```python
from build123d import *

# Parameters (mm, degrees)
F1_DEPTH = 3.5
F2_R     = 10
F3_DEPTH = 3.501
F4_R     = 12
F4_R_2   = 10
F5_DEPTH = 25
F6_SIZE  = 1.5


with BuildPart() as f1:
    # F0 (on Top) → F1 (new body)
    with BuildSketch(Plane.XY):
        with BuildLine():
            ThreePointArc((102.5, 82.5), (96.6421356237, 96.6421356237), (82.5, 102.5))
            Line((82.5, 102.5), (-82.5, 102.5))
            ThreePointArc((-82.5, 102.5), (-96.6421356237, 96.6421356237), (-102.5, 82.5))
            Line((-102.5, 82.5), (-102.5, -82.5))
            ThreePointArc((-102.5, -82.5), (-96.6421356237, -96.6421356237), (-82.5, -102.5))
            Line((-82.5, -102.5), (82.5, -102.5))
            ThreePointArc((82.5, -102.5), (96.6421356237, -96.6421356237), (102.5, -82.5))
            Line((102.5, -82.5), (102.5, 82.5))
        make_face()
    extrude(amount=F1_DEPTH)

    # F2 (on Top) → F3 (cut, through all)
    with BuildSketch(Plane.XY):
        with Locations((-78, 78)):
            Circle(F2_R)
        with Locations((-78, 39)):
            Circle(F2_R)
        with Locations((-78, 0)):
            Circle(F2_R)
        with Locations((-78, -39)):
            Circle(F2_R)
        with Locations((-78, -78)):
            Circle(F2_R)
        with Locations((-39, 78)):
            Circle(F2_R)
        with Locations((-39, 39)):
            Circle(F2_R)
        with Locations((-39, 0)):
            Circle(F2_R)
        with Locations((-39, -39)):
            Circle(F2_R)
        with Locations((-39, -78)):
            Circle(F2_R)
        with Locations((0, 78)):
            Circle(F2_R)
        with Locations((0, 39)):
            Circle(F2_R)
        Circle(F2_R)
        with Locations((0, -39)):
            Circle(F2_R)
        with Locations((0, -78)):
            Circle(F2_R)
        with Locations((39, 78)):
            Circle(F2_R)
        with Locations((39, 39)):
            Circle(F2_R)
        with Locations((39, 0)):
            Circle(F2_R)
        with Locations((39, -39)):
            Circle(F2_R)
        with Locations((39, -78)):
            Circle(F2_R)
        with Locations((78, 78)):
            Circle(F2_R)
        with Locations((78, 39)):
            Circle(F2_R)
        with Locations((78, 0)):
            Circle(F2_R)
        with Locations((78, -39)):
            Circle(F2_R)
        with Locations((78, -78)):
            Circle(F2_R)
    extrude(amount=F3_DEPTH, mode=Mode.SUBTRACT)

    # F4 (on face) → F5 (join)
    with BuildSketch(Plane(origin=(0, 0, 0), x_dir=(1, 0, 0), z_dir=(0, 0, -1))):
        with Locations((-78, -78)):
            Circle(F4_R)
        with Locations((-78, -78)):
            Circle(F4_R_2, mode=Mode.SUBTRACT)
        with Locations((-78, 0)):
            Circle(F4_R)
        with Locations((-78, 0)):
            Circle(F4_R_2, mode=Mode.SUBTRACT)
        with Locations((-78, 78)):
            Circle(F4_R)
        with Locations((-78, 78)):
            Circle(F4_R_2, mode=Mode.SUBTRACT)
        with Locations((0, -78)):
            Circle(F4_R)
        with Locations((0, -78)):
            Circle(F4_R_2, mode=Mode.SUBTRACT)
        Circle(F4_R)
        Circle(F4_R_2, mode=Mode.SUBTRACT)
        with Locations((0, 78)):
            Circle(F4_R)
        with Locations((0, 78)):
            Circle(F4_R_2, mode=Mode.SUBTRACT)
        with Locations((78, -78)):
            Circle(F4_R)
        with Locations((78, -78)):
            Circle(F4_R_2, mode=Mode.SUBTRACT)
        with Locations((78, 0)):
            Circle(F4_R)
        with Locations((78, 0)):
            Circle(F4_R_2, mode=Mode.SUBTRACT)
        with Locations((78, 78)):
            Circle(F4_R)
        with Locations((78, 78)):
            Circle(F4_R_2, mode=Mode.SUBTRACT)
    extrude(amount=F5_DEPTH)

    # F6
    f6_edges = [f1.edges().sort_by_distance(p)[0] for p in [
        (96.642136, 96.642136, 3.5),
        (102.5, 0, 3.5),
        (0, 102.5, 3.5),
        (96.642136, -96.642136, 3.5),
        (-96.642136, 96.642136, 3.5),
        (0, -102.5, 3.5),
        (-102.5, 0, 3.5),
        (-96.642136, -96.642136, 3.5),
        (-88, -78, 3.5),
        (-49, -78, 3.5),
        (-88, -39, 3.5),
        (-49, -39, 3.5),
        (-10, -78, 3.5),
        (29, -78, 3.5),
        (68, -78, 3.5),
        (-10, -39, 3.5),
        (29, -39, 3.5),
        (68, -39, 3.5),
        (-88, 0, 3.5),
        (-88, 39, 3.5),
        (-49, 0, 3.5),
        (-49, 39, 3.5),
        (-88, 78, 3.5),
        (-49, 78, 3.5),
        (-10, 0, 3.5),
        (29, 0, 3.5),
        (-10, 39, 3.5),
        (29, 39, 3.5),
        (68, 0, 3.5),
        (68, 39, 3.5),
        (-10, 78, 3.5),
        (29, 78, 3.5),
        (68, 78, 3.5),
    ]]
    chamfer(f6_edges, length=F6_SIZE)


solid = f1.part
```
CAD build for the part. Positions are in the model's coordinates, mm. A direction names the side the tool comes from. Round coordinates to 2 decimals unless told otherwise and drop trailing zeros. Write each loop counter-clockwise with the first axis right and the second up, starting at its lowest first coordinate (ties: lowest second). Pieces come first, ordered by that corner, then holes. Notation, with made-up numbers: (1, -15.5) - (24, -15.5) arc R24 ccw to (24, -5.5) - close; hole circle Ø8 at (8, 47). An arc over 180 degrees is marked (long way). Write item = value, one per line. Start each with the question number.
Q1. Drop flat-ended pins along their axis: pin 1 (18 mm diameter, centred on x = -78, y = -78, fed in from +Z); pin 2 (8 mm diameter, centred on x = -7, z = -5, fed in from -Y); pin 3 (1 mm diameter, centred on x = -62, y = 0, fed in from -Z). Give the stop position or say it passes through.
Q2. Which spindle directions (+Z, -Z, +X, -X, +Y, -Y) get a long thin tool onto all of the face, cutting with end or side? Do faces 3 (the cylindrical face through (-1.302, 87.915, -11.689)), 4 (the cylindrical face through (-89.99, -0.53, -12.32)). Say none if no direction does.
Q3. Probe L1, parallel to X at y = 0, z = -11.5; L2, parallel to Y at x = 0, z = 1.05. List the from-to ranges inside material, lowest first. Write a range as from..to.
Q4. Band-saw the part on A-A (z = -6). Count the separate pieces of the cut face and the enclosed holes in it, then the cut area to 3 significant figures.
Q5. Mould opens along Y. For faces 1 (the cylindrical face through (-96.486, 96.797, 0.986)), 2 (the cylindrical face through (70.63, 84.76, -11.69)) say: pulls with the +Y half, pulls with the -Y half, needs draft (parallel to the pull), parting line crosses it, or undercut.
Q6. Band-saw the part on C-C (x = -24). Give the cut face in (y, z).
Answers below:
q1.pin_1 = through
q1.pin_2 = -89.62
q1.pin_3 = 0
q2.face_3 = +Z, -Z
q2.face_4 = -Z
q3.L1 = -90..-88, -68..-66, -12..-10, 10..12, 66..68, 88..90
q3.L2 = -102.5..-88, -68..-49, -29..-10, 10..29, 49..68, 88..102.5
q4.separate_pieces = 9
q4.enclosed_holes = 9
q4.area = 1,240 mm2
q5.face_1 = pulls with the +Y half
q5.face_2 = undercut
q6.outline = (-102.5, 0) - (102.5, 0) - (102.5, 2) - (101, 3.5) - (-101, 3.5) - (-102.5, 2) - close
